Read the model definition and answer for the solid it produces. Units are mm, in the model's axes. A direction names the side the tool comes from. Give positions to 0.01 mm unless a question says otherwise; leave off trailing zeros. Write each loop counter-clockwise with the first axis right and the second up, starting at its lowest first coordinate (ties: lowest second). Pieces come first, ordered by that corner, then holes. Notation, with made-up numbers: M 29.5,25 L 69.5,25 A25 ccw 69.5,50 Z; hole C -9,-31 d10. An arc over 180 degrees is marked long. Use a Markdown table: item, result. Add a question column.
Item 1: The mould has two halves that part along Z. Classify faces 5 (the flat face through (-20, 3, 20.2)), 6 (the flat face through (0, 0, 0)), 7 (the flat face through (1, 5.2, -10)): pulls with the +Z half, pulls with the -Z half, needs draft (parallel to the pull), parting line crosses it, or undercut.
Item 2: For faces 1 (the flat face through (1, 5.2, 10)), 2 (the cylindrical face through (-22.452, 3.579, 19.355)), 3 (the flat face through (18.35, 3, 17)), 4 (the flat face through (1, 3, -11.2)), determine the directions among +Z, -Z, +X, -X, +Y, -Y from which every point of the face is accessible in a straight line to the end or side of a thin tool.
Item 3: Given P1, Ø1.1, axis at x = -8.5, y = 5.5, coming from the +Z side; P2, Ø1.9, axis at y = 2, z = 9, coming from the -X side; P3, Ø1.9, axis at y = 3.5, z = 15.5, coming from the +X side, each flat-ended and moving along its own axis, determine where each tip first touches the part or whether it passes through.
Item 4: A cutting plane is placed at B-B on x = -14. Determine the outline of the cut face in (y, z).
Item 5: Consider probe 1 along Z at (x, y) = (-17, 5); probe 2 along X at (y, z) = (5.75, 17); probe 3 along X at (y, z) = (3.25, 18.5). Determine where each line is inside the solid, lowest interval first. Write a range as [from, to].
Item 6: A cutting plane is placed at C-C on y = 0.5. Determine the outline of the cut face in (x, z), then the cut area to 3 significant figures.
Item 7: A cutting plane is placed at A-A on z = 18.2. Determine the outline of the cut face in (x, y), then the cut area to 4 significant figures.
Autodesk Inventor part; units mm, degrees
ref_plane "YZ Plane" through (0, 0, 0) normal (1, 0, 0) x (0, 1, 0)
ref_plane "XZ Plane" through (0, 0, 0) normal (0, 1, 0) x (-1, 0, 0)
ref_plane "XY Plane" through (0, 0, 0) normal (0, 0, 1) x (1, 0, 0)
sketch "Skizze1" plane through (0, 0, 0) normal (0, 1, 0) x (-1, 0, 0)
  line L0 (-20.85, 11.2) -> (18.85, 11.2)
  line L1 (18.85, 11.2) -> (18.85, -11.2)
  line L2 (18.85, -11.2) -> (-20.85, -11.2)
  line L3 (-20.85, -11.2) -> (-20.85, 11.2)
  line L4 (-20.85, 11.2) -> (18.85, -11.2) construction
  line L5 (18.85, 11.2) -> (-20.85, -11.2) construction
  point P0 (0, 0)
  point P1 (-1, 0)
  dimension "d24" = 39.7
  dimension "d25" = 22.4
  dimension "d26" = 1
  dimension "d27" = 0
extrude "Extrusion1" add sketch "Skizze1" along normal blind 1
sketch "Skizze2" plane through (0, 0, 0) normal (0, 1, 0) x (-1, 0, 0)
  line L0 (-20.85, 11.2) -> (-20.85, -11.2)
  line L1 (18.85, 11.2) -> (-20.85, 11.2)
  line L2 (20.85, -13.2) -> (-20.85, -13.2)
  line L3 (-20.85, -13.2) -> (-20.85, 13.2)
  line L4 (-20.85, 13.2) -> (20.85, 13.2)
  line L5 (20.85, 13.2) -> (20.85, -13.2)
  line L6 (20.85, -13.2) -> (-20.85, 13.2) construction
  line L7 (-20.85, -13.2) -> (20.85, 13.2) construction
  line L8 (18.85, -11.2) -> (18.85, 11.2)
  line L9 (-20.85, 11.2) -> (18.85, 11.2)
  line L10 (18.85, 11.2) -> (18.85, -11.2)
  line L11 (18.85, -11.2) -> (-20.85, -11.2)
  point P0 (0, 0)
  dimension "d30" = 2
  dimension "d31" = 2
extrude "Extrusion2" add sketch "Skizze2" along normal blind 5.2 contours L3 L4 L5 L2 L11 L8 L1
sketch "Skizze3" plane through (0, 5.2, 0) normal (0, 1, 0) x (1, 0, 0)
  line L0 (20.85, 13.2) -> (-20.85, 13.2)
  line L1 (20.85, -13.2) -> (20.85, 13.2)
  line L2 (-20.85, 13.2) -> (20.85, 13.2)
  line L3 (20.85, 13.2) -> (20.85, -13.2)
  line L4 (20.85, -13.2) -> (-20.85, -13.2)
  line L5 (-20.85, -13.2) -> (-20.85, 13.2)
  line L6 (-20.85, 13.2) -> (20.85, -13.2) construction
  line L7 (20.85, 13.2) -> (-20.85, -13.2) construction
  line L8 (20.85, -11.2) -> (20.85, 11.2)
  line L9 (20.85, 9.2) -> (20.85, -9.2)
  line L10 (20.85, -11.2) -> (-18.85, -11.2)
  line L11 (-18.85, 11.2) -> (20.85, 11.2)
  line L12 (-18.85, -11.2) -> (-18.85, 11.2)
  line L13 (20.85, -9.2) -> (-18.85, -9.2)
  line L14 (-18.85, 9.2) -> (20.85, 9.2)
  point P0 (0, 0)
  point P1 (20.85, -9.2)
  dimension "d35" = 2
  dimension "d36" = 2
extrude "Extrusion3" add sketch "Skizze3" along normal blind 1 contours L1 L11 L12 L10 L4 L5 L0 | L1 L14 L12 L11 | L1 L10 L12 L13
sketch "Skizze7" plane through (20.85, 1, 11.2) normal (0, 0, -1) x (-1, 0, 0)
  line L0 (39.7, 4.2) -> (0, 4.2) construction
  line L1 (3.25, 4.2) -> (3.25, 0) construction
  line L2 (0, 0) -> (39.7, 0) construction
  line L3 (0, -1) -> (0, 5.2) construction
  circle A0 centre (3.25, 2.1) radius 0.75
  point P0 (20.85, -1)
  dimension "d38" = 1.5
  dimension "d39" = 2.5
extrude "Extrusion7" add sketch "Skizze7" along normal blind 0.3 draft -50
mirror "Spiegeln2" about plane through (0, 0, 0) normal (0, 0, 1) of "Extrusion7"
sketch "Skizze8" plane through (-20.85, 0, 13.2) normal (0, 0, 1) x (1, 0, 0)
  line L0 (0, 0) -> (0, 6.2)
  line L1 (41.7, 6.2) -> (2, 6.2)
  line L2 (0, 0) -> (2.5, 0)
  line L3 (2.5, 0) -> (2.5, 6.2)
  line L4 (2.5, 6.2) -> (0, 6.2)
  line L5 (0, 6.2) -> (0, 0)
  point P0 (20.85, 0)
  dimension "d42" = 2.5
extrude "Extrusion8" add sketch "Skizze8" along normal blind 7
sketch "Skizze9" plane through (-20.85, 0, -13.2) normal (-1, 0, 0) x (0, 0, 1)
  line L0 (26.4, 6.2) -> (33.4, 6.2) construction
  line L1 (31.4, 6.2) -> (31.4, 0) construction
  line L2 (33.4, 6.2) -> (33.4, 0) construction
  circle A0 centre (31.4, 3.1) radius 1.25
  point P0 (13.2, 0)
  dimension "d45" = 2
  dimension "d46" = 2.5
extrude "Extrusion9" add sketch "Skizze9" along normal blind 3.25
mirror "Spiegeln3" about plane through (0, 0, 0) normal (1, 0, 0) of "Extrusion8", "Extrusion9"
sketch "Skizze10" plane through (-20.85, 0, -13.2) normal (-1, 0, 0) x (0, 0, 1)
  line L0 (26.4, 6.2) -> (26.4, 0)
  line L1 (26.4, 6.2) -> (26.4, 0)
  line L2 (0, 0) -> (33.4, 0)
  circle A0 centre (31.4, 3.1) radius 1.25
  point P0 (13.2, 0)
  dimension "d49" = 3.75
properties part number "CaseV1"
Filled in:
| question | item | result |
|---|---|---|
| 1 | face 5 | pulls with the +Z half |
| 1 | face 6 | needs draft |
| 1 | face 7 | undercut |
| 2 | face 1 | +X |
| 2 | face 2 | -X |
| 2 | face 3 | +Z, +Y, -Y |
| 2 | face 4 | none |
| 3 | P1 | z = 13.2 |
| 3 | P2 | x = -20.85 |
| 3 | P3 | x = 20.85 |
| 4 | outline | M 0,-13.2 L 6.2,-13.2 L 6.2,-9.2 L 5.2,-9.2 L 5.2,-11.2 L 1,-11.2 L 1,11.2 L 5.2,11.2 L 5.2,9.2 L 6.2,9.2 L 6.2,13.2 L 0,13.2 Z |
| 5 | probe 1 | [-13.2, -11.2], [11.2, 13.2] |
| 5 | probe 2 | [-20.85, -18.35], [18.35, 20.85] |
| 5 | probe 3 | [-24.1, -18.35], [18.35, 24.1] |
| 6 | outline | M -20.85,-13.2 L 20.85,-13.2 L 20.85,20.2 L 18.35,20.2 L 18.35,13.2 L -18.35,13.2 L -18.35,20.2 L -20.85,20.2 Z |
| 6 | area | 1,140 mm² |
| 7 | outline | M -24.1,1.85 L -20.85,1.85 L -20.85,0 L -18.35,0 L -18.35,6.2 L -20.85,6.2 L -20.85,4.35 L -24.1,4.35 Z; M 18.35,0 L 20.85,0 L 20.85,1.85 L 24.1,1.85 L 24.1,4.35 L 20.85,4.35 L 20.85,6.2 L 18.35,6.2 Z |
| 7 | area | 47.25 mm² |
